from build123d import *

# Parameters (mm, degrees)
F1_DEPTH = 5
F0_W     = 4
F0_H     = 9.65
F2_DEPTH = 5
F3_SIZE2 = 5
F3_SIZE  = 1.5
F4_SIZE2 = 1.5
F4_SIZE  = 5
F0_W_2   = 1.575


with BuildPart() as f1:
    # F0 (on Front) → F1 (new body, symmetric)
    with BuildSketch(Plane.XZ):
        Polygon((-4.6942626456, -1.1915529846), (-4.6942626456, -4.1915529846), (1.8057373544, -4.1915529846), (1.8057373544, 5.4584470154), (-4.6942626456, 5.4584470154), (-4.6942626456, 2.4584470154), (-1.6942626456, 2.4584470154), (-1.6942626456, -1.1915529846), align=None)
    extrude(amount=F1_DEPTH, both=True)

    # F0 (on Front) → F2 (join, symmetric)
    with BuildSketch(Plane.XZ):
        with Locations((3.8057373544, 0.6334470154)):
            Rectangle(F0_W, F0_H)
    extrude(amount=F2_DEPTH, both=True)

    # F3
    f3_edges = [f1.edges().sort_by_distance(p)[0] for p in [
        (5.805737, -5, 0.633447),
    ]]
    f3_side = f1.faces().sort_by_distance((5.805737, 0, 0.633447))[0]
    chamfer(f3_edges, length=F3_SIZE, length2=F3_SIZE2, reference=f3_side)

    # F4
    f4_edges = [f1.edges().sort_by_distance(p)[0] for p in [
        (5.805737, 5, 0.633447),
    ]]
    f4_side = f1.faces().sort_by_distance((1.010094, 5, 0.633447))[0]
    chamfer(f4_edges, length=F4_SIZE, length2=F4_SIZE2, reference=f4_side)

    # F0 (on Front) → F5 (revolve, cut)
    with BuildSketch(Plane.XZ):
        with Locations((6.5932373544, 0.6334470154)):
            Rectangle(F0_W_2, F0_H)
    revolve(axis=Axis((5.8057373544, 0, 0.6334470154), (0, 0, -1)), mode=Mode.SUBTRACT)

    # F0 (on Front) → F6 (revolve)
    with BuildSketch(Plane.XZ):
        Polygon((7.3807373544, 5.4584470154), (7.3807373544, -4.1915529846), (9.3057373544, -4.159483593), (9.3057373544, 5.4584470154), align=None)
    revolve(axis=Axis((5.8057373544, 0, 0.6334470154), (0, 0, -1)))


solid = f1.part
The listing builds one solid part. Answer for the finished solid, in the listing's coordinates (mm). A direction names the side the tool comes from. Coordinates: 2 decimals unless noted, no trailing zeros. Order: outer loops, then holes, each group sorted by start corner. A loop starts at its lowest first (then second) coordinate and runs counter-clockwise, first axis right, second up. Notation, with made-up numbers: (-34.75, 35) -> (5.25, 35) arc R32 cw to (5.25, 68) -> close; hole circle Ø11 at (66, -6.75). An arc over 180 degrees is marked (long way). Answer in a Markdown table with one row per item. Add a question column.
Item 1: Find the intervals of material crossed by L1, parallel to X at y = 0, z = 2.5; L2, parallel to Z at x = -1.75, y = -4.25; L3, parallel to X at y = 0, z = 0, in increasing order. Write a range as from..to.
Item 2: This flat-tipped pin is pushed along its axis until it touches: P1, Ø3, axis at y = 3.5, z = -1.5, coming from the +X side. Where does it stop, or does it pass through?
Item 3: Which of the six approach directions +Z, -Z, +X, -X, +Y, -Y give full straight-line access (tool end or side, diameter ignored) to faces 1 (the face through (-3, 0, -1.192)), 2 (the face through (4.232, -0.069, 0.566)), 3 (the face through (7.715, 0.042, -4.186))?
Item 4: Find section A-A (y = 0). Write down the section's boundary in (x, z), then the cut area to 3 significant figures.
Item 5: Find section C-C (x = 4.75). Write down the section's boundary in (y, z), then the cut area to 3 significant figures.
Item 6: Determine the mould class of faces 4 (the face through (-4.694, 0, 4)), 5 (the face through (-3, 0, 2.458)), 6 (the face through (0, 0, -4.192)) for opening direction Z: +Z half, -Z half, draft (parallel to the pull), parting line (faces both ways), or undercut.
Item 7: Find section B-B (z = 2). Write down the section's boundary in (x, y) (3 decimals), then the cut area to 3 significant figures.
Result set:
| question | item | result |
|---|---|---|
| 1 | L1 | x = -4.69..4.23, 7.38..9.31 |
| 1 | L2 | z = -4.19..-1.19, 2.46..5.46 |
| 1 | L3 | x = -1.69..4.23, 7.38..9.31 |
| 2 | P1 | stops at x = 8.68 |
| 3 | face 1 | -X, +Y, -Y |
| 3 | face 2 | +Z, -Z |
| 3 | face 3 | -Z, +X |
| 4 | outline | (-4.69, -4.19) -> (4.23, -4.19) -> (4.23, 5.46) -> (-4.69, 5.46) -> (-4.69, 2.46) -> (-1.69, 2.46) -> (-1.69, -1.19) -> (-4.69, -1.19) -> close; (7.38, -4.19) -> (9.31, -4.16) -> (9.31, 5.46) -> (7.38, 5.46) -> close |
| 4 | area | 93.7 mm² |
| 5 | outline | (-3.82, -4.19) -> (-1.17, -4.19) -> (-1.17, 5.46) -> (-3.82, 5.46) -> close; (1.17, -4.19) -> (3.82, -4.19) -> (3.82, 5.46) -> (1.17, 5.46) -> close |
| 5 | area | 51.1 mm² |
| 6 | face 4 | draft |
| 6 | face 5 | undercut |
| 6 | face 6 | -Z half |
| 7 | outline | (-1.694, -5) -> (0.806, -5) -> (5.806, -3.5) arc R3.5 ccw to (5.806, 3.5) -> (0.806, 5) -> (-1.694, 5) -> close; hole circle Ø3.15 at (5.806, 0) |
| 7 | area | 78.9 mm² |
